from build123d import *

# Parameters (mm, degrees)
SKETCH1_W                  = 100
SKETCH1_H                  = 135
STOCK_DEPTH                = 3
BASE_ROUNDS_R              = 4
SKETCH2_R                  = 1.75
HOLES_LAYERS_DEPTH         = 85.055041491
SKETCH4_R                  = 1.5
HOLES_INTERFACEBOARD_DEPTH = 85.055041491
SKETCH3_R                  = 1.25
HOLES_MOTORBRACKET_DEPTH   = 85.055041491
HOLES_MOTORWIRES_DEPTH     = 85.055041491
SKETCH5_R                  = 2.25
HOLES_BALLCASTER_DEPTH     = 85.055041491
SKETCH6_R                  = 1.5
HOLES_COLOR_IRSENSOR_DEPTH = 85.055041491
STRAPHOLE_POWERBANK_DEPTH  = 85.055041491
SKETCH7_R                  = 1.5
HOLES_PI_DEPTH             = 85.055041491
SKETCH10_R                 = 1.5
HOLES_DCDC_DEPTH           = 85.055041491
SKETCH13_R                 = 1.5
HOLES_IMU_DEPTH            = 85.055041491


with BuildPart() as part:
    # Sketch1 → Stock (new body)
    with BuildSketch(Plane(origin=(0, 0, 0), x_dir=(1, 0, 0), z_dir=(0, 1, 0))):
        Rectangle(SKETCH1_W, SKETCH1_H)
    extrude(amount=-STOCK_DEPTH)

    # base-rounds
    base_rounds_edges = [part.edges().sort_by_distance(p)[0] for p in [
        (50, -1.5, 67.5),
        (-50, -1.5, 67.5),
        (-50, -1.5, -67.5),
        (50, -1.5, -67.5),
    ]]
    fillet(base_rounds_edges, radius=BASE_ROUNDS_R)

    # Sketch2 → holes-layers (cut, through all)
    with BuildSketch(Plane(origin=(0, 0, 0), x_dir=(1, 0, 0), z_dir=(0, 1, 0))):
        with Locations(Location((-44, -61.5, 0), (0, 0, 270))):
            Circle(SKETCH2_R)
        with Locations(Location((-44, 61.5, 0), (0, 0, 90))):
            Circle(SKETCH2_R)
        with Locations(Location((44, -61.5, 0), (0, 0, 90))):
            Circle(SKETCH2_R)
        with Locations(Location((44, 61.5, 0), (0, 0, 270))):
            Circle(SKETCH2_R)
        with Locations(Location((-37, -14.5, 0), (0, 0, 270))):
            Circle(SKETCH2_R)
        with Locations(Location((37, -14.5, 0), (0, 0, 90))):
            Circle(SKETCH2_R)
    extrude(amount=-HOLES_LAYERS_DEPTH, mode=Mode.SUBTRACT)

    # Sketch4 → holes-interfaceboard (cut, through all)
    with BuildSketch(Plane(origin=(0, 0, 0), x_dir=(1, 0, 0), z_dir=(0, 1, 0))):
        with Locations(Location((-38, -63.5, 0), (0, 0, 270))):
            Circle(SKETCH4_R)
        with Locations(Location((-38, -47.5, 0), (0, 0, 270))):
            Circle(SKETCH4_R)
        with Locations(Location((38, -47.5, 0), (0, 0, 90))):
            Circle(SKETCH4_R)
        with Locations(Location((38, -63.5, 0), (0, 0, 90))):
            Circle(SKETCH4_R)
    extrude(amount=-HOLES_INTERFACEBOARD_DEPTH, mode=Mode.SUBTRACT)

    # Sketch3 → holes-motorbracket (cut, through all)
    with BuildSketch(Plane(origin=(0, 0, 0), x_dir=(1, 0, 0), z_dir=(0, 1, 0))):
        with Locations(Location((-45, -35.5, 0), (0, 0, 270))):
            Circle(SKETCH3_R)
        with Locations(Location((-45, -17.5, 0), (0, 0, 270))):
            Circle(SKETCH3_R)
        with Locations(Location((45, -17.5, 0), (0, 0, 270))):
            Circle(SKETCH3_R)
        with Locations(Location((45, -35.5, 0), (0, 0, 270))):
            Circle(SKETCH3_R)
    extrude(amount=-HOLES_MOTORBRACKET_DEPTH, mode=Mode.SUBTRACT)

    # Sketch11 → holes-motorwires (cut, through all)
    with BuildSketch(Plane(origin=(0, 0, 0), x_dir=(1, 0, 0), z_dir=(0, 1, 0))):
        with BuildLine():
            Line((-34, -20), (-28, -20))
            ThreePointArc((-28, -20), (-27.292893219, -20.292893219), (-27, -21))
            Line((-27, -21), (-27, -32))
            ThreePointArc((-27, -32), (-27.292893219, -32.707106781), (-28, -33))
            Line((-28, -33), (-34, -33))
            ThreePointArc((-34, -33), (-34.707106781, -32.707106781), (-35, -32))
            Line((-35, -32), (-35, -21))
            ThreePointArc((-35, -21), (-34.707106781, -20.292893219), (-34, -20))
        make_face()
        with BuildLine():
            Line((27, -21), (27, -32))
            ThreePointArc((27, -32), (27.292893219, -32.707106781), (28, -33))
            Line((28, -33), (34, -33))
            ThreePointArc((34, -33), (34.707106781, -32.707106781), (35, -32))
            Line((35, -32), (35, -21))
            ThreePointArc((35, -21), (34.707106781, -20.292893219), (34, -20))
            Line((34, -20), (28, -20))
            ThreePointArc((28, -20), (27.292893219, -20.292893219), (27, -21))
        make_face()
    extrude(amount=-HOLES_MOTORWIRES_DEPTH, mode=Mode.SUBTRACT)

    # Sketch5 → holes-ballcaster (cut, through all)
    with BuildSketch(Plane(origin=(0, 0, 0), x_dir=(1, 0, 0), z_dir=(0, 1, 0))):
        with Locations(Location((-19.35, 47.5, 0), (0, 0, 270))):
            Circle(SKETCH5_R)
        with Locations(Location((19.35, 47.5, 0), (0, 0, 270))):
            Circle(SKETCH5_R)
    extrude(amount=-HOLES_BALLCASTER_DEPTH, mode=Mode.SUBTRACT)

    # Sketch6 → holes-color_irsensor (cut, through all)
    with BuildSketch(Plane(origin=(0, 0, 0), x_dir=(1, 0, 0), z_dir=(0, 1, 0))):
        with Locations(Location((-7.62, -62.5, 0), (0, 0, 270))):
            Circle(SKETCH6_R)
        with Locations(Location((7.62, -62.5, 0), (0, 0, 270))):
            Circle(SKETCH6_R)
    extrude(amount=-HOLES_COLOR_IRSENSOR_DEPTH, mode=Mode.SUBTRACT)

    # Sketch8 → straphole-powerbank (cut, through all)
    with BuildSketch(Plane(origin=(0, 0, 0), x_dir=(1, 0, 0), z_dir=(0, 1, 0))):
        with BuildLine():
            Line((-15.5, -9.5), (-13.5, -9.5))
            ThreePointArc((-13.5, -9.5), (-12.792893219, -9.792893219), (-12.5, -10.5))
            Line((-12.5, -10.5), (-12.5, -19.5))
            ThreePointArc((-12.5, -19.5), (-12.792893219, -20.207106781), (-13.5, -20.5))
            Line((-13.5, -20.5), (-26.5, -20.5))
            ThreePointArc((-26.5, -20.5), (-27.207106781, -20.207106781), (-27.5, -19.5))
            Line((-27.5, -19.5), (-27.5, -10.5))
            ThreePointArc((-27.5, -10.5), (-27.207106781, -9.792893219), (-26.5, -9.5))
            Line((-26.5, -9.5), (-24.5, -9.5))
            ThreePointArc((-24.5, -9.5), (-23.792893219, -9.792893219), (-23.5, -10.5))
            Line((-23.5, -10.5), (-23.5, -13.5))
            Line((-23.5, -13.5), (-24.25, -13.5))
            ThreePointArc((-24.25, -13.5), (-24.426776695, -13.573223305), (-24.5, -13.75))
            Line((-24.5, -13.75), (-24.5, -15.5))
            ThreePointArc((-24.5, -15.5), (-24.207106781, -16.207106781), (-23.5, -16.5))
            Line((-23.5, -16.5), (-16.5, -16.5))
            ThreePointArc((-16.5, -16.5), (-15.792893219, -16.207106781), (-15.5, -15.5))
            Line((-15.5, -15.5), (-15.5, -13.75))
            ThreePointArc((-15.5, -13.75), (-15.573223305, -13.573223305), (-15.75, -13.5))
            Line((-15.75, -13.5), (-16.5, -13.5))
            Line((-16.5, -13.5), (-16.5, -10.5))
            ThreePointArc((-16.5, -10.5), (-16.207106781, -9.792893219), (-15.5, -9.5))
        make_face()
        with BuildLine():
            Line((15.5, -15.5), (15.5, -13.75))
            ThreePointArc((15.5, -13.75), (15.573223305, -13.573223305), (15.75, -13.5))
            Line((15.75, -13.5), (16.5, -13.5))
            Line((16.5, -13.5), (16.5, -10.5))
            ThreePointArc((16.5, -10.5), (16.207106781, -9.792893219), (15.5, -9.5))
            Line((15.5, -9.5), (13.5, -9.5))
            ThreePointArc((13.5, -9.5), (12.792893219, -9.792893219), (12.5, -10.5))
            Line((12.5, -10.5), (12.5, -19.5))
            ThreePointArc((12.5, -19.5), (12.792893219, -20.207106781), (13.5, -20.5))
            Line((13.5, -20.5), (26.5, -20.5))
            ThreePointArc((26.5, -20.5), (27.207106781, -20.207106781), (27.5, -19.5))
            Line((27.5, -19.5), (27.5, -10.5))
            ThreePointArc((27.5, -10.5), (27.207106781, -9.792893219), (26.5, -9.5))
            Line((26.5, -9.5), (24.5, -9.5))
            ThreePointArc((24.5, -9.5), (23.792893219, -9.792893219), (23.5, -10.5))
            Line((23.5, -10.5), (23.5, -13.5))
            Line((23.5, -13.5), (24.25, -13.5))
            ThreePointArc((24.25, -13.5), (24.426776695, -13.573223305), (24.5, -13.75))
            Line((24.5, -13.75), (24.5, -15.5))
            ThreePointArc((24.5, -15.5), (24.207106781, -16.207106781), (23.5, -16.5))
            Line((23.5, -16.5), (16.5, -16.5))
            ThreePointArc((16.5, -16.5), (15.792893219, -16.207106781), (15.5, -15.5))
        make_face()
        with BuildLine():
            Line((-15.5, 66.5), (-15.5, 64.75))
            ThreePointArc((-15.5, 64.75), (-15.573223305, 64.573223305), (-15.75, 64.5))
            Line((-15.75, 64.5), (-16.5, 64.5))
            Line((-16.5, 64.5), (-16.5, 61.5))
            ThreePointArc((-16.5, 61.5), (-16.207106781, 60.792893219), (-15.5, 60.5))
            Line((-15.5, 60.5), (-13.5, 60.5))
            ThreePointArc((-13.5, 60.5), (-12.792893219, 60.792893219), (-12.5, 61.5))
            Line((-12.5, 61.5), (-12.5, 70.5))
            ThreePointArc((-12.5, 70.5), (-12.792893219, 71.207106781), (-13.5, 71.5))
            Line((-13.5, 71.5), (-26.5, 71.5))
            ThreePointArc((-26.5, 71.5), (-27.207106781, 71.207106781), (-27.5, 70.5))
            Line((-27.5, 70.5), (-27.5, 61.5))
            ThreePointArc((-27.5, 61.5), (-27.207106781, 60.792893219), (-26.5, 60.5))
            Line((-26.5, 60.5), (-24.5, 60.5))
            ThreePointArc((-24.5, 60.5), (-23.792893219, 60.792893219), (-23.5, 61.5))
            Line((-23.5, 61.5), (-23.5, 64.5))
            Line((-23.5, 64.5), (-24.25, 64.5))
            ThreePointArc((-24.25, 64.5), (-24.426776695, 64.573223305), (-24.5, 64.75))
            Line((-24.5, 64.75), (-24.5, 66.5))
            ThreePointArc((-24.5, 66.5), (-24.207106781, 67.207106781), (-23.5, 67.5))
            Line((-23.5, 67.5), (-16.5, 67.5))
            ThreePointArc((-16.5, 67.5), (-15.792893219, 67.207106781), (-15.5, 66.5))
        make_face()
        with BuildLine():
            Line((15.5, 60.5), (13.5, 60.5))
            ThreePointArc((13.5, 60.5), (12.792893219, 60.792893219), (12.5, 61.5))
            Line((12.5, 61.5), (12.5, 70.5))
            ThreePointArc((12.5, 70.5), (12.792893219, 71.207106781), (13.5, 71.5))
            Line((13.5, 71.5), (26.5, 71.5))
            ThreePointArc((26.5, 71.5), (27.207106781, 71.207106781), (27.5, 70.5))
            Line((27.5, 70.5), (27.5, 61.5))
            ThreePointArc((27.5, 61.5), (27.207106781, 60.792893219), (26.5, 60.5))
            Line((26.5, 60.5), (24.5, 60.5))
            ThreePointArc((24.5, 60.5), (23.792893219, 60.792893219), (23.5, 61.5))
            Line((23.5, 61.5), (23.5, 64.5))
            Line((23.5, 64.5), (24.25, 64.5))
            ThreePointArc((24.25, 64.5), (24.426776695, 64.573223305), (24.5, 64.75))
            Line((24.5, 64.75), (24.5, 66.5))
            ThreePointArc((24.5, 66.5), (24.207106781, 67.207106781), (23.5, 67.5))
            Line((23.5, 67.5), (16.5, 67.5))
            ThreePointArc((16.5, 67.5), (15.792893219, 67.207106781), (15.5, 66.5))
            Line((15.5, 66.5), (15.5, 64.75))
            ThreePointArc((15.5, 64.75), (15.573223305, 64.573223305), (15.75, 64.5))
            Line((15.75, 64.5), (16.5, 64.5))
            Line((16.5, 64.5), (16.5, 61.5))
            ThreePointArc((16.5, 61.5), (16.207106781, 60.792893219), (15.5, 60.5))
        make_face()
    extrude(amount=-STRAPHOLE_POWERBANK_DEPTH, mode=Mode.SUBTRACT)

    # Sketch7 → holes-pi (cut, through all)
    with BuildSketch(Plane(origin=(0, 0, 0), x_dir=(1, 0, 0), z_dir=(0, 1, 0))):
        with Locations(Location((-29, -64.5, 0), (0, 0, 270))):
            Circle(SKETCH7_R)
        with Locations(Location((-29, -41.5, 0), (0, 0, 270))):
            Circle(SKETCH7_R)
        with Locations(Location((29, -64.5, 0), (0, 0, 90))):
            Circle(SKETCH7_R)
        with Locations(Location((29, -41.5, 0), (0, 0, 90))):
            Circle(SKETCH7_R)
    extrude(amount=-HOLES_PI_DEPTH, mode=Mode.SUBTRACT)

    # Sketch10 → holes-dcdc (cut, through all)
    with BuildSketch(Plane(origin=(0, 0, 0), x_dir=(1, 0, 0), z_dir=(0, 1, 0))):
        with Locations(Location((-15.25, -23.5, 0), (0, 0, 270))):
            Circle(SKETCH10_R)
        with Locations(Location((15.25, -39.5, 0), (0, 0, 90))):
            Circle(SKETCH10_R)
        with Locations(Location((-15.25, -39.5, 0), (0, 0, 270))):
            Circle(SKETCH10_R)
        with Locations(Location((15.25, -23.5, 0), (0, 0, 270))):
            Circle(SKETCH10_R)
    extrude(amount=-HOLES_DCDC_DEPTH, mode=Mode.SUBTRACT)

    # Sketch13 → holes-IMU (cut, through all)
    with BuildSketch(Plane(origin=(0, 0, 0), x_dir=(1, 0, 0), z_dir=(0, 1, 0))):
        with Locations(Location((-10.44998, -29.12, 0), (0, 0, 270))):
            Circle(SKETCH13_R)
        with Locations(Location((10.44998, -29.12, 0), (0, 0, 90))):
            Circle(SKETCH13_R)
    extrude(amount=-HOLES_IMU_DEPTH, mode=Mode.SUBTRACT)


solid = part.part
Can you work these out from the model? Positions are in its coordinate system, mm. A direction names the side the tool comes from. Coordinates: 2 decimals unless noted, no trailing zeros. Order: outer loops, then holes, each group sorted by start corner. A loop starts at its lowest first (then second) coordinate and runs counter-clockwise, first axis right, second up. Notation, with made-up numbers: (-15, 40) -> (-9, 40) arc R12 ccw to (-9, 51) -> close; hole circle Ø4 at (27, -30). An arc over 180 degrees is marked (long way). Use one line per item in the form item = value.
Q1. I need wall thicknesses on L1, parallel to X at y = -1.15, z = 31; L2, parallel to X at y = -1.8, z = -47.5; L3, parallel to Z at x = 25.5, y = -0.25. Which ranges of each line are inside material? Lowest first, please.
From the geometry:
L1 = -50 to -35, -27 to 27, 35 to 50
L2 = -50 to -21.6, -17.1 to 17.1, 21.6 to 50
L3 = -60.5 to 9.5, 20.5 to 67.5
Q2. Which directions (+Z, -Z, +X, -X, +Y, -Y) give clear straight access to the entire face, cutting with the end or side of a thin tool? Please do faces 4 (the face through (-1, -3, -1)), 5 (the face through (-27.5, -1, 15)).
From the geometry:
face_4 = +Z, -Z, +X, -X, -Y
face_5 = +Y, -Y
Q3. Imagine slicing it at C-C, the plane y = -2.1. Give the number of separate pieces and of enclosed holes in the cut face, then the cut area to 3 significant figures.
From the geometry:
separate_pieces = 1
enclosed_holes = 32
area = 12,700 mm²
Q4. Will these pins go through, and if not, where does the flat tip stop? P1, Ø4, axis at x = -45, z = 17.5, coming from the +Y side; P2, Ø0.6, axis at x = -14.5, y = -1.5, coming from the -Z side.
From the geometry:
P1 = 0
P2 = -60.5
Q5. Imagine slicing it at B-B, the plane x = -19.35. List the corners of the cut face in (y, z) for me, then the cut area to 4 significant figures.
From the geometry:
outline = (-3, -67.5) -> (0, -67.5) -> (0, -49.75) -> (-3, -49.75) -> close; (-3, -45.25) -> (0, -45.25) -> (0, 16.5) -> (-3, 16.5) -> close; (-3, 20.5) -> (0, 20.5) -> (0, 67.5) -> (-3, 67.5) -> close
area = 379.5 mm²
Q6. We'd pull the mould along X, two halves only. Please class faces 1 (the face through (-1, -1, 67.5)), 2 (the face through (-43.33, -1.479, -63.117)), 3 (the face through (48.859, -1.521, -66.297)): released by +X, released by -X, zero draft, split by the parting line, or undercut.
From the geometry:
face_1 = zero draft
face_2 = undercut
face_3 = released by +X
Q7. Imagine slicing it at A-A, the plane z = -47.5. List the corners of the cut face in (x, y) for me.
From the geometry:
outline = (-50, -3) -> (-21.6, -3) -> (-21.6, 0) -> (-50, 0) -> close; (-17.1, -3) -> (17.1, -3) -> (17.1, 0) -> (-17.1, 0) -> close; (21.6, -3) -> (50, -3) -> (50, 0) -> (21.6, 0) -> close
